Geometry check sheet. Reference: the model listing, model coordinates, mm. Round coordinates to 2 decimals unless told otherwise and drop trailing zeros. Write each loop counter-clockwise with the first axis right and the second up, starting at its lowest first coordinate (ties: lowest second). Pieces come first, ordered by that corner, then holes. Notation, with made-up numbers: M 6,4.5 L 57,4.5 A30 ccw 57,43.5 Z; hole C 73.25,-28 d4. An arc over 180 degrees is marked long. Use a Markdown table: item, result.
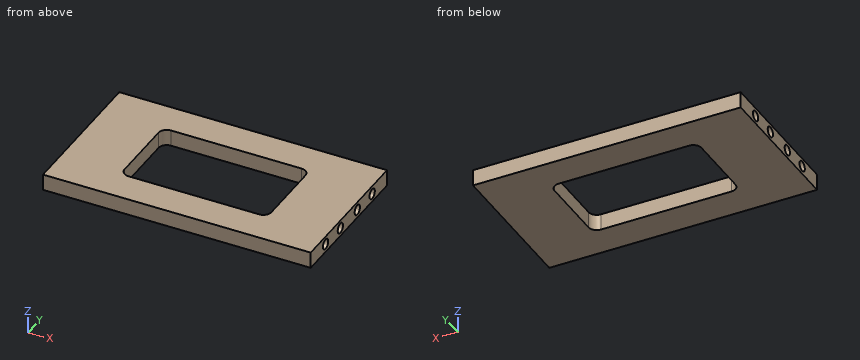
Autodesk Inventor part; units mm, degrees
ref_plane "YZ Plane" through (0, 0, 0) normal (1, 0, 0) x (0, 1, 0)
ref_plane "XZ Plane" through (0, 0, 0) normal (0, 1, 0) x (-1, 0, 0)
ref_plane "XY Plane" through (0, 0, 0) normal (0, 0, 1) x (1, 0, 0)
sketch "스케치1" plane through (0, 0, 0) normal (0, 0, 1) x (1, 0, 0)
  line L0 (-32.8, 18) -> (32.8, 18)
  line L1 (32.8, 18) -> (32.8, -18)
  line L2 (32.8, -18) -> (-32.8, -18)
  line L3 (-32.8, -18) -> (-32.8, 18)
  line L4 (-32.8, 18) -> (32.8, -18) construction
  line L5 (32.8, 18) -> (-32.8, -18) construction
  point P0 (0, 0)
  dimension "d0" = 65.6
  dimension "d1" = 36
extrude "돌출1" add sketch "스케치1" along normal blind 4
sketch "스케치2" plane through (32.8, -18, 0) normal (1, 0, 0) x (0, 0, -1)
  line L0 (0, 0) -> (0, 36)
  line L1 (0, 36) -> (-4, 36)
  line L2 (-4, 0) -> (-4, 36)
  line L3 (0, 0) -> (-4, 0)
  line L4 (0, 0) -> (-4, 0)
  line L5 (-2, 0) -> (-2, 36) construction
  line L6 (0, 36) -> (-4, 36)
  circle A0 centre (-2, 7) radius 1.25
  circle A1 centre (-2, 14) radius 1.25
  circle A2 centre (-2, 22) radius 1.25
  circle A3 centre (-2, 29) radius 1.25
  point P0 (0, 18)
  dimension "d4" = 2.5
  dimension "d5" = 2.5
  dimension "d7" = 2.5
  dimension "d8" = 7
  dimension "d9" = 7
  dimension "d11" = 2.5
  dimension "d12" = 7
  dimension "d13" = 7
extrude "돌출2" cut sketch "스케치2" against normal blind 6 contours A0 | A1 | A2 | A3
mirror "미러1" about plane through (0, 0, 0) normal (1, 0, 0) of "돌출2"
sketch "스케치3" plane through (0, 0, 4) normal (0, 0, 1) x (1, 0, 0)
  line L0 (18, -10) -> (-18, -10)
  line L1 (-18, -10) -> (-18, 10)
  line L2 (-18, 10) -> (18, 10)
  line L3 (18, 10) -> (18, -10)
  line L4 (18, -10) -> (-18, 10) construction
  line L5 (-18, -10) -> (18, 10) construction
  point P0 (0, 0)
  dimension "d16" = 36
  dimension "d17" = 20
extrude "돌출3" cut sketch "스케치3" against normal blind 6
fillet "모깎기1" radius 2 4 edges at (18, -10, 2) (18, 10, 2) (-18, 10, 2) (-18, -10, 2)
properties part number "지지프레임1" material "알루미늄 6061"
Item 1: Material ranges on line 1 along Y through (x, z) = (29, 2); line 2 along X through (y, z) = (3.5, 0.4); line 3 along X through (y, z) = (-4, 2.7), recorded low to high. Write a range as from..to.
Outcome:
| item | result |
|---|---|
| line 1 | y = -18..-12.25, -9.75..-5.25, -2.75..2.75, 5.25..9.75, 12.25..18 |
| line 2 | x = -32.8..-18, 18..32.8 |
| line 3 | x = -26.8..-18, 18..26.8 |
Item 2: Cross-section at A-A, the plane y = -4. Record the cut outline in (x, z).
Outcome:
| item | result |
|---|---|
| outline | M -32.8,0 L -18,0 L -18,4 L -32.8,4 L -32.8,3.25 L -26.8,3.25 L -26.8,0.75 L -32.8,0.75 Z; M 18,0 L 32.8,0 L 32.8,0.75 L 26.8,0.75 L 26.8,3.25 L 32.8,3.25 L 32.8,4 L 18,4 Z |
Item 3: Cross-section at D-D, the plane y = 0. Record the cut outline in (x, z), and give its area (3 significant figures).
Outcome:
| item | result |
|---|---|
| outline | M -32.8,0 L -18,0 L -18,4 L -32.8,4 Z; M 18,0 L 32.8,0 L 32.8,4 L 18,4 Z |
| area | 118 mm2 |
Item 4: Go/stop test with flat-tipped pins: pin 1 (2 mm diameter, centred on y = -11, z = 2, fed in from +X); pin 2 (2 mm diameter, centred on y = -4, z = 2, fed in from -X). Record where each tip stops, or that it passes through.
Outcome:
| item | result |
|---|---|
| pin 1 | stops at x = 26.8 |
| pin 2 | stops at x = -26.8 |
Item 5: Cross-section at C-C, the plane y = -11. Record the cut outline in (x, z), and give its area (3 significant figures).
Outcome:
| item | result |
|---|---|
| outline | M -32.8,0 L 32.8,0 L 32.8,0.75 L 26.8,0.75 L 26.8,3.25 L 32.8,3.25 L 32.8,4 L -32.8,4 L -32.8,3.25 L -26.8,3.25 L -26.8,0.75 L -32.8,0.75 Z |
| area | 232 mm2 |
Item 6: Cross-section at B-B, the plane x = 14. Record the cut outline in (y, z).
Outcome:
| item | result |
|---|---|
| outline | M -18,0 L -10,0 L -10,4 L -18,4 Z; M 10,0 L 18,0 L 18,4 L 10,4 Z |
